```python
from build123d import *

# Parameters (mm, degrees)
SKETCH1_R           = 17.5
SKETCH1_R_2         = 2
BOSS_EXTRUDE1_DEPTH = 4
SKETCH2_R           = 8
BOSS_EXTRUDE2_DEPTH = 17
SKETCH3_R           = 5.5
CUT_EXTRUDE1_DEPTH  = 12
SKETCH4_R           = 6
CUT_EXTRUDE2_DEPTH  = 1.1
SKETCH5_R           = 5.5
CUT_EXTRUDE3_DEPTH  = 2.9
SKETCH6_R           = 2.75
CUT_EXTRUDE4_DEPTH  = 5.5


with BuildPart() as part:
    # Sketch1 → Boss-Extrude1 (new body)
    with BuildSketch(Plane(origin=(0, 0, 0), x_dir=(1, 0, 0), z_dir=(0, 1, 0))):
        with Locations(Location((0, 0, 0), (0, 0, 270))):
            Circle(SKETCH1_R)
        with Locations(Location((0, 13, 0), (0, 0, 270))):
            Circle(SKETCH1_R_2, mode=Mode.SUBTRACT)
        with Locations(Location((13, 0, 0), (0, 0, 270))):
            Circle(SKETCH1_R_2, mode=Mode.SUBTRACT)
        with Locations(Location((0, -13, 0), (0, 0, 270))):
            Circle(SKETCH1_R_2, mode=Mode.SUBTRACT)
        with Locations(Location((-13, 0, 0), (0, 0, 270))):
            Circle(SKETCH1_R_2, mode=Mode.SUBTRACT)
    extrude(amount=BOSS_EXTRUDE1_DEPTH)

    # Sketch2 → Boss-Extrude2 (add)
    with BuildSketch(Plane.XZ):
        with Locations(Location((0, 0, 0), (0, 0, 270))):
            Circle(SKETCH2_R)
    extrude(amount=BOSS_EXTRUDE2_DEPTH)

    # Sketch3 → Cut-Extrude1 (cut)
    with BuildSketch(Plane(origin=(0, 4, 0), x_dir=(1, 0, 0), z_dir=(0, 1, 0))):
        with Locations(Location((0, 0, 0), (0, 0, 270))):
            Circle(SKETCH3_R)
    extrude(amount=-CUT_EXTRUDE1_DEPTH, mode=Mode.SUBTRACT)

    # Sketch4 → Cut-Extrude2 (cut)
    with BuildSketch(Plane(origin=(0, -8, 0), x_dir=(1, 0, 0), z_dir=(0, 1, 0))):
        with Locations(Location((0, 0, 0), (0, 0, 270))):
            Circle(SKETCH4_R)
    extrude(amount=-CUT_EXTRUDE2_DEPTH, mode=Mode.SUBTRACT)

    # Sketch5 → Cut-Extrude3 (cut)
    with BuildSketch(Plane(origin=(0, -9.1, 0), x_dir=(1, 0, 0), z_dir=(0, 1, 0))):
        with Locations(Location((0, 0, 0), (0, 0, 270))):
            Circle(SKETCH5_R)
    extrude(amount=-CUT_EXTRUDE3_DEPTH, mode=Mode.SUBTRACT)

    # Sketch6 → Cut-Extrude4 (cut)
    with BuildSketch(Plane.XZ.offset(17)):
        with Locations(Location((0, 0, 0), (0, 0, 270))):
            Circle(SKETCH6_R)
    extrude(amount=-CUT_EXTRUDE4_DEPTH, mode=Mode.SUBTRACT)


solid = part.part
```
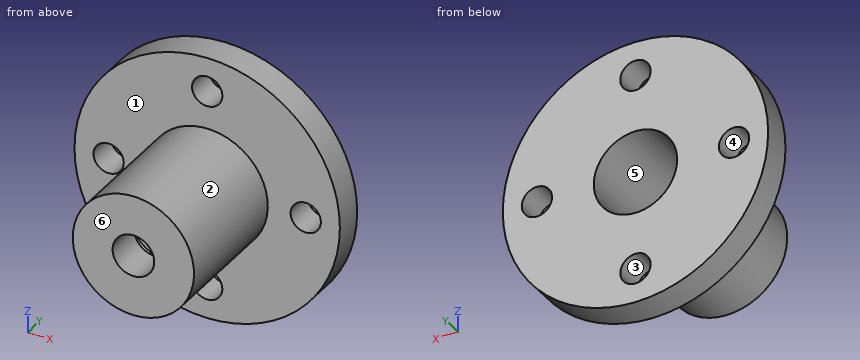
The listing builds one solid part. Answer for the finished solid, in the listing's coordinates (mm). Face numbers are marked on the shaded views. A direction names the side the tool comes from. Round coordinates to 2 decimals unless told otherwise and drop trailing zeros. Loops run counter-clockwise (first coordinate to the right, second up) from the corner with the lowest first, then second, coordinate; pieces in that order, holes last. Notation, with made-up numbers: (70, 47.25) - (81, 47.25) arc R23 cw to (81, 61.25) - close; hole circle Ø2 at (-2.75, 50). An arc over 180 degrees is marked (long way). Use one line per item in the form item = value. Start each with the question number.
1. For a pull along Z with two mould halves and no side action, classify the marked faces 1, 2, 3 and 4 as pulls with the +Z half, pulls with the -Z half, needs draft (parallel to the pull), parting line crosses it, or undercut.
2. The part is cut by section D-D on z = 12.5. Determine the outline of the cut face in (x, y), then the cut area to 3 significant figures.
3. A tool of negligible diameter and unlimited length cuts with its end or side. For the marked faces 5 and 6, from which of +Z, -Z, +X, -X, +Y, -Y can it reach the whole face along a straight path? Write none if from no direction.
4. Given pin 1 Ø10 at (x, y) = (1.5, -12) entering from +Z; pin 2 Ø1 at (y, z) = (-9.5, 0.5) entering from -X; pin 3 Ø2 at (y, z) = (-4.5, 6) entering from +X (3 decimals), each flat-ended and moving along its own axis, determine where each tip first touches the part or whether it passes through.
5. The part is cut by section C-C on y = -4. Determine the outline of the cut face in (x, z), then the cut area to 3 significant figures.
6. The part is cut by section B-B on x = 13.5. Determine the outline of the cut face in (y, z).
7. The part is cut by section A-A on z = 0. Give the number of separate pieces and of enclosed holes in the cut face, then the cut area to 3 significant figures.
8. Consider line 1 (X direction, y = 1.5, z = 0); line 2 (Y direction, x = 1.5, z = -11.5); line 3 (X direction, y = -10.5, z = 0). Determine where each line is inside the solid, lowest interval first. Write a range as [from, to].
Geometry check:
q1.face_1 = needs draft
q1.face_2 = parting line crosses it
q1.face_3 = undercut
q1.face_4 = undercut
q2.outline = (-12.25, 0) - (-1.94, 0) - (-1.94, 4) - (-12.25, 4) - close; (1.94, 0) - (12.25, 0) - (12.25, 4) - (1.94, 4) - close
q2.area = 82.5 mm^2
q3.face_5 = +Y
q3.face_6 = +Z, -Z, +X, -X, -Y
q4.pin_1 = 8
q4.pin_2 = -8
q4.pin_3 = 6.245
q5.outline = circle Ø16 at (0, 0); hole circle Ø11 at (0, 0)
q5.area = 106 mm^2
q6.outline = (0, -11.14) - (4, -11.14) - (4, -1.94) - (0, -1.94) - close; (0, 1.94) - (4, 1.94) - (4, 11.14) - (0, 11.14) - close
q7.separate_pieces = 4
q7.enclosed_holes = 0
q7.area = 175 mm^2
q8.line_1 = [-17.5, -15], [-11, -5.5], [5.5, 11], [15, 17.5]
q8.line_2 = [0, 4]
q8.line_3 = [-8, -5.5], [5.5, 8]
